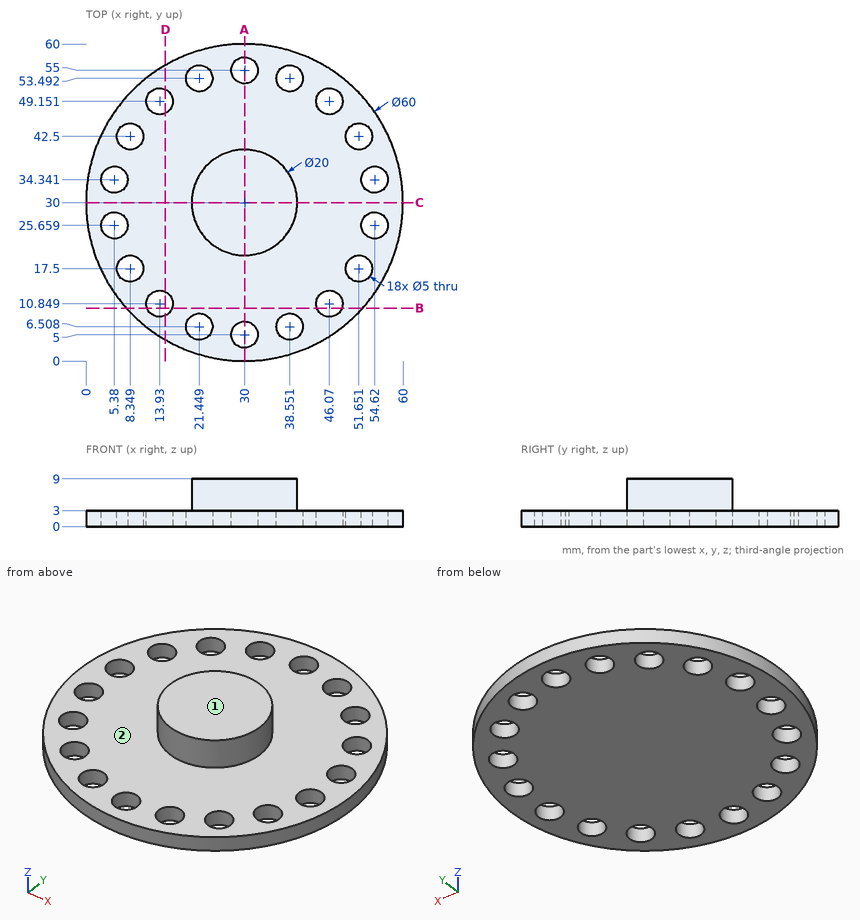
Job drawing, mm, ordinate dimensions from the low corner. One solid piece. A direction names the side the tool comes from. Coordinates: 2 decimals unless noted, no trailing zeros. Write each loop counter-clockwise with the first axis right and the second up, starting at its lowest first coordinate (ties: lowest second). Pieces come first, ordered by that corner, then holes.
Item 1: Slice it at D-D (x = 15). Write the cut outline in (y, z).
Item 2: Which spindle directions (+Z, -Z, +X, -X, +Y, -Y) get a long thin tool onto all of the face, cutting with end or side? Do the marked faces 1 and 2. Say none if no direction does.
Item 3: Slice it at A-A (x = 30). Write the cut outline in (y, z), and give its area (3 significant figures).
Item 4: Pin check, flat tips, straight feed: pin 1 (8 mm diameter, centred on x = 13.93, y = 10.85, fed in from +Z); pin 2 (1.5 mm diameter, centred on x = 24, z = 7, fed in from +Y); pin 3 (5 mm diameter, centred on y = 52, z = 3.5, fed in from -X) (1 decimal). Stop position of each tip, or through.
Item 5: Slice it at C-C (y = 30). Write the cut outline in (x, z), and give its area (3 significant figures).
Item 6: Slice it at B-B (y = 10). Write the cut outline in (x, z).
Item 7: Probe line 1 (X direction, y = 54, z = 2) (1 decimal); line 2 (Y direction, x = 52, z = 1.75) (1 decimal); line 3 (Z direction, x = 38.5, y = 23.5). List the from-to ranges inside material, lowest first.
Results found:
1. outline: (4.02, 0) - (8.59, 0) - (8.59, 3) - (4.02, 3) - close; (13.11, 0) - (46.89, 0) - (46.89, 3) - (13.11, 3) - close; (51.41, 0) - (55.98, 0) - (55.98, 3) - (51.41, 3) - close
2. face 1: +Z, +X, -X, +Y, -Y
2. face 2: +Z
3. outline: (0, 0) - (2.5, 0) - (2.5, 3) - (0, 3) - close; (7.5, 0) - (52.5, 0) - (52.5, 3) - (40, 3) - (40, 9) - (20, 9) - (20, 3) - (7.5, 3) - close; (57.5, 0) - (60, 0) - (60, 3) - (57.5, 3) - close
3. area: 270 mm2
4. pin 1: stops at z = 3
4. pin 2: stops at y = 38.51
4. pin 3: stops at x = 7.2
5. outline: (0, 0) - (60, 0) - (60, 3) - (40, 3) - (40, 9) - (20, 9) - (20, 3) - (0, 3) - close
5. area: 300 mm2
6. outline: (7.64, 0) - (11.58, 0) - (11.58, 3) - (7.64, 3) - close; (16.28, 0) - (43.72, 0) - (43.72, 3) - (16.28, 3) - close; (48.42, 0) - (52.36, 0) - (52.36, 3) - (48.42, 3) - close
7. line 1: x = 12 to 19, 23.9 to 27.7, 32.3 to 36.1, 41 to 48
7. line 2: y = 9.6 to 15, 20 to 40, 45 to 50.4
7. line 3: z = 0 to 3
